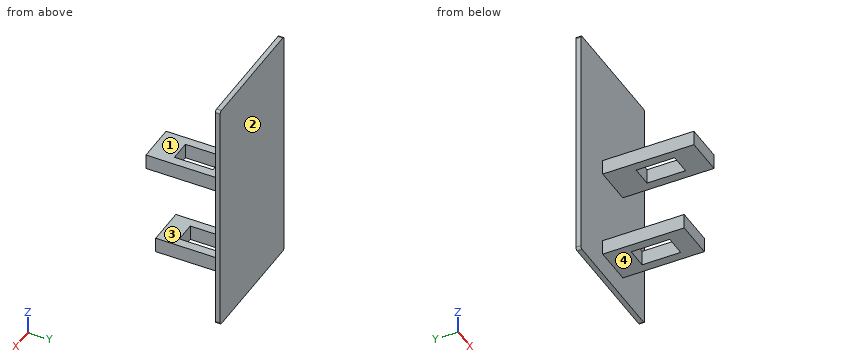
Autodesk Inventor part; units mm, degrees
ref_plane "to_base_XY" through (0, 0, 0) normal (0, 1, 0) x (1, 0, 0)
ref_plane "to_base_YZ" through (0, 0, 0) normal (1, 0, 0) x (0, 0, -1)
ref_plane "to_base_ZX" through (0, 0, 0) normal (0, 0, -1) x (0, 1, 0)
sketch "Sketch_2" plane through (0, 0, 0) normal (0, 1, 0) x (-1, 0, 0)
  line L0 (3.1877, -6.1184) -> (3.1877, 6.1184)
  arc A0 (3.1877, 6.1184) -> (3.0577, 6.2484) centre (3.0577, 6.1184) ccw
  line L1 (3.0577, 6.2484) -> (-3.0577, 6.2484)
  arc A1 (-3.0577, 6.2484) -> (-3.1877, 6.1184) centre (-3.0577, 6.1184) ccw
  line L2 (-3.1877, 6.1184) -> (-3.1877, -6.1184)
  arc A2 (-3.1877, -6.1184) -> (-3.0577, -6.2484) centre (-3.0577, -6.1184) ccw
  line L3 (-3.0577, -6.2484) -> (3.0577, -6.2484)
  arc A3 (3.0577, -6.2484) -> (3.1877, -6.1184) centre (3.0577, -6.1184) ccw
extrude "Extrusion1" add sketch "Sketch_2" along normal blind 0.254
sketch "Sketch_12" plane through (0, 0, -4.699) normal (0, 0, 1) x (1, 0, 0)
  line L0 (-1.0033, 0) -> (-1.0033, -4.2418)
  line L1 (-1.0033, -4.2418) -> (1.0033, -4.2418)
  line L2 (1.0033, -4.2418) -> (1.0033, 0)
  line L3 (1.0033, 0) -> (-1.0033, 0)
  line L4 (-0.5461, -1.2446) -> (-0.5461, -3.2512)
  line L5 (-0.5461, -3.2512) -> (0.5461, -3.2512)
  line L6 (0.5461, -3.2512) -> (0.5461, -1.2446)
  line L7 (0.5461, -1.2446) -> (-0.5461, -1.2446)
extrude "Extrusion2" add sketch "Sketch_12" along normal mid plane 0.7874
sketch "Sketch_14" plane through (0, 0, 0) normal (0, 0, 1) x (1, 0, 0)
  line L0 (-1.0033, 0) -> (-1.0033, -4.7498)
  line L1 (-1.0033, -4.7498) -> (1.0033, -4.7498)
  line L2 (1.0033, -4.7498) -> (1.0033, 0)
  line L3 (1.0033, 0) -> (-1.0033, 0)
  line L4 (-0.5461, -1.4986) -> (-0.5461, -3.5052)
  line L5 (-0.5461, -3.5052) -> (0.5461, -3.5052)
  line L6 (0.5461, -3.5052) -> (0.5461, -1.4986)
  line L7 (0.5461, -1.4986) -> (-0.5461, -1.4986)
extrude "Extrusion3" add sketch "Sketch_14" along normal mid plane 0.7874
ref_plane "to_base_XY" through (0, 0, 0) normal (0, 1, 0) x (1, 0, 0)
ref_plane "to_base_YZ" through (0, 0, 0) normal (1, 0, 0) x (0, 0, -1)
ref_plane "to_base_ZX" through (0, 0, 0) normal (0, 0, -1) x (0, 1, 0)
properties part number "M201101-terminals"
CAD build for the part. Positions are in the model's coordinates, mm. Face numbers are marked on the shaded views. Give positions to 0.01 mm unless a question says otherwise; leave off trailing zeros. Order: outer loops, then holes, each group sorted by start corner. A loop starts at its lowest first (then second) coordinate and runs counter-clockwise, first axis right, second up.
(1) Flat gauge pins, fed straight in: pin 1 (3 mm diameter, centred on x = 0, y = -4, fed in from +Z); pin 2 (1.9 mm diameter, centred on x = 1, z = 2, fed in from -Y); pin 3 (0.9 mm diameter, centred on y = -1.5, z = 0, fed in from +X). Where does each tip first touch, or does it go through?
(2) Drill centre lines: L1, parallel to Z at x = -0.75, y = -3.9; L2, parallel to Y at x = 1, z = -2. Where is each one in solid material? Low to high.
(3) Saw through at B-B, the plane y = -2. Give the cut face in (x, z), then the cut area to 3 significant figures.
(4) Saw through at A-A, the plane x = 0. Give the cut face in (y, z).
(5) Saw through at C-C, the plane y = -0.9. Give the cut face in (x, z).
(6) Saw through at D-D, the plane z = 0. Give the cut face in (x, y).
(7) Mould opens along Z. For the marked faces 1, 2, 3 and 4 say: released by +Z, released by -Z, zero draft, split by the parting line, or undercut.
Results found:
1. pin 1: stops at z = 0.39
1. pin 2: stops at y = 0
1. pin 3: stops at x = 1
2. L1: z = -5.09 to -4.31, -0.39 to 0.39
2. L2: y = 0 to 0.25
3. outline: (-1, -5.09) - (-0.55, -5.09) - (-0.55, -4.31) - (-1, -4.31) - close; (-1, -0.39) - (-0.55, -0.39) - (-0.55, 0.39) - (-1, 0.39) - close; (0.55, -5.09) - (1, -5.09) - (1, -4.31) - (0.55, -4.31) - close; (0.55, -0.39) - (1, -0.39) - (1, 0.39) - (0.55, 0.39) - close
3. area: 1.44 mm2
4. outline: (-4.75, -0.39) - (-3.51, -0.39) - (-3.51, 0.39) - (-4.75, 0.39) - close; (-4.24, -5.09) - (-3.25, -5.09) - (-3.25, -4.31) - (-4.24, -4.31) - close; (-1.5, -0.39) - (0, -0.39) - (0, -4.31) - (-1.24, -4.31) - (-1.24, -5.09) - (0, -5.09) - (0, -6.25) - (0.25, -6.25) - (0.25, 6.25) - (0, 6.25) - (0, 0.39) - (-1.5, 0.39) - close
5. outline: (-1, -5.09) - (1, -5.09) - (1, -4.31) - (-1, -4.31) - close; (-1, -0.39) - (1, -0.39) - (1, 0.39) - (-1, 0.39) - close
6. outline: (-3.19, 0) - (-1, 0) - (-1, -4.75) - (1, -4.75) - (1, 0) - (3.19, 0) - (3.19, 0.25) - (-3.19, 0.25) - close; hole (-0.55, -3.51) - (0.55, -3.51) - (0.55, -1.5) - (-0.55, -1.5) - close
7. face 1: released by +Z
7. face 2: zero draft
7. face 3: undercut
7. face 4: released by -Z
